Could you check a few things on this drawing? It's one solid part, dimensions in mm from its lowest x, y, z. Give positions to 0.01 mm unless a question says otherwise; leave off trailing zeros. Loops run counter-clockwise (first coordinate to the right, second up) from the corner with the lowest first, then second, coordinate; pieces in that order, holes last. Notation, with made-up numbers: (66.5, -0.75) - (111.5, -0.75) arc R15 cw to (111.5, 16.25) - close; hole circle Ø3 at (-3, 9). An arc over 180 degrees is marked (long way). Write item = value, one per line.
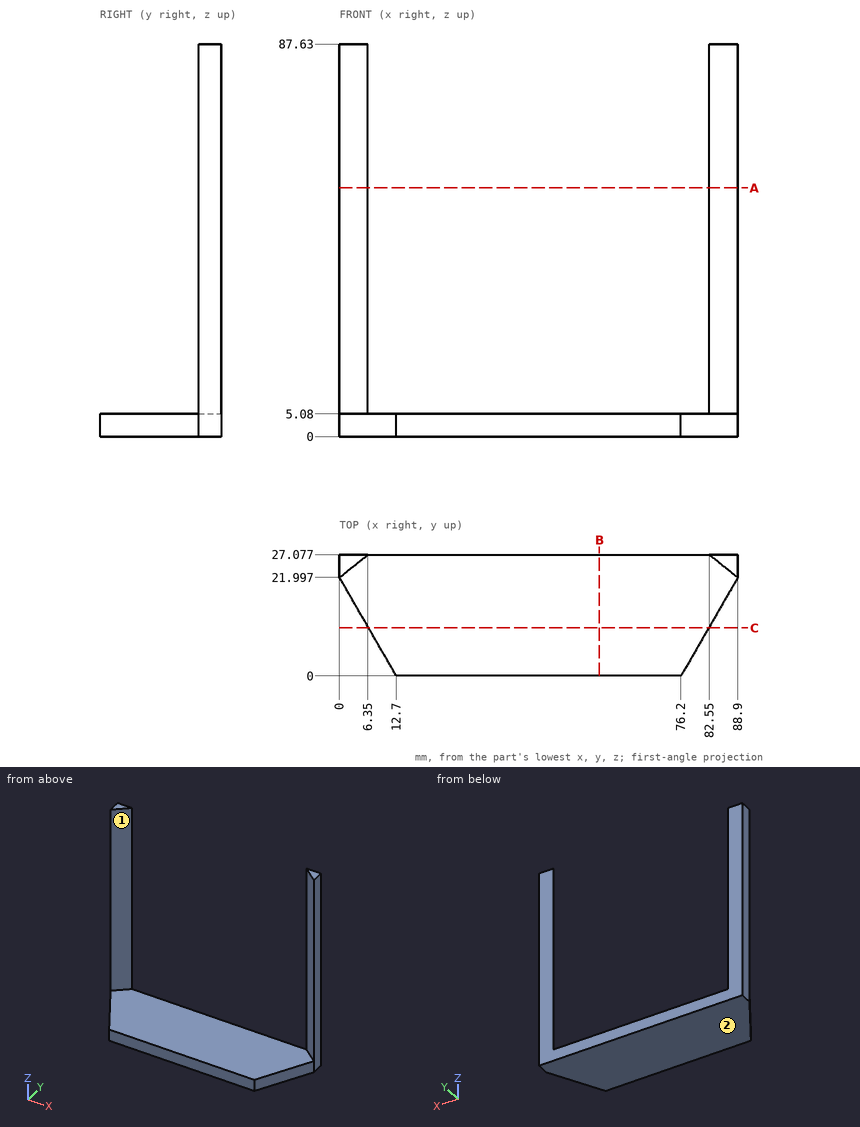
Q1. We'd pull the mould along X, two halves only. Please class the marked faces 1 and 2: released by +X, released by -X, zero draft, split by the parting line, or undercut.
Output:
face_1 = undercut
face_2 = zero draft
Q2. I need wall thicknesses on L1, parallel to Z at x = 69.5, y = 18.5; L2, parallel to X at y = 24.25, z = 60.5; L3, parallel to X at y = 25.75, z = 56.5. Which ranges of each line are inside material? Lowest first, please.
Output:
L1 = 0 to 5.08
L2 = 0 to 2.82, 86.08 to 88.9
L3 = 0 to 4.69, 84.21 to 88.9
Q3. Imagine slicing it at C-C, the plane y = 10.75. Write out the boundary of the cut face in (x, z), then the cut area to 3 significant figures.
Output:
outline = (6.49, 0) - (82.41, 0) - (82.41, 5.08) - (6.49, 5.08) - close
area = 386 mm2
Q4. Imagine slicing it at B-B, the plane x = 58. Write out the boundary of the cut face in (y, z), then the cut area to 3 significant figures.
Output:
outline = (0, 0) - (27.08, 0) - (27.08, 5.08) - (0, 5.08) - close
area = 138 mm2
Q5. Imagine slicing it at A-A, the plane z = 55.5. Write out the boundary of the cut face in (x, y), then the cut area to 3 significant figures.
Output:
outline = (0, 22) - (6.35, 27.08) - (0, 27.08) - close; (82.55, 27.08) - (88.9, 22) - (88.9, 27.08) - close
area = 32.3 mm2
Q6. For pin 1 (10 mm diameter, centred on x = 33, y = 19, fed in from +Z); pin 2 (3 mm diameter, centred on x = 9.5, z = 13.5, fed in from -Y), each with a flat end and sliding along its axis, tell me the tip position at first contact or that it passes through.
Output:
pin_1 = 5.08
pin_2 = through
